Work out the finished part from the listing and answer in its coordinate system (mm). Face numbers are marked on the shaded views. Coordinates: 2 decimals unless noted, no trailing zeros. Loops run counter-clockwise (first coordinate to the right, second up) from the corner with the lowest first, then second, coordinate; pieces in that order, holes last. Notation, with made-up numbers: M -25.75,89 L 21.25,89 A16 ccw 21.25,105 Z; hole C 59,70 d5. An arc over 180 degrees is marked long. Write each question's results on one line, items separated by ' | '.
```python
from build123d import *

# Parameters (mm, degrees)
F1_DEPTH = 7
F2_DEPTH = 5
F3_W     = 25.4
F3_H     = 7
F4_DEPTH = 19.05
F6_DEPTH = 7


with BuildPart() as f1:
    # F0 (on Top) → F1 (new body)
    with BuildSketch(Plane.XY):
        with BuildLine():
            ThreePointArc((20, 20), (40, 0), (20, -20))
            Line((20, -20), (-40, -20))
            Line((-40, -20), (-40, -45.4))
            Line((-40, -45.4), (20, -45.4))
            ThreePointArc((20, -45.4), (65.4, 0), (20, 45.4))
            Line((20, 45.4), (-40, 45.4))
            Line((-40, 45.4), (-40, 20))
            Line((-40, 20), (20, 20))
        make_face()
        with BuildLine():
            Line((-40, -20), (20, -20))
            ThreePointArc((20, -20), (40, 0), (20, 20))
            Line((20, 20), (-40, 20))
            Line((-40, 20), (-40, -20))
        make_face()
    extrude(amount=F1_DEPTH)

    # F0 (on Top) → F2 (cut)
    with BuildSketch(Plane.XY):
        with BuildLine():
            Line((-40, -20), (20, -20))
            ThreePointArc((20, -20), (40, 0), (20, 20))
            Line((20, 20), (-40, 20))
            Line((-40, 20), (-40, -20))
        make_face()
    extrude(amount=F2_DEPTH, mode=Mode.SUBTRACT)

    # F3 (on face) → F4 (join)
    with BuildSketch(Plane(origin=(-40, 0, 0), x_dir=(0, -1, 0), z_dir=(-1, 0, 0))):
        with Locations((-32.7, 3.5)):
            Rectangle(F3_W, F3_H)
        with Locations((32.7, 3.5)):
            Rectangle(F3_W, F3_H)
    extrude(amount=F4_DEPTH)

    # F5 (on face) → F6 (join, through all)
    with BuildSketch(Plane(origin=(0, 0, 0), x_dir=(1, 0, 0), z_dir=(0, 0, -1))):
        with BuildLine():
            Line((-59.05, -65.72), (20, -65.72))
            ThreePointArc((20, -65.72), (85.72, 0), (20, 65.72))
            Line((20, 65.72), (-59.05, 65.72))
            Line((-59.05, 65.72), (-59.05, 45.4))
            Line((-59.05, 45.4), (20, 45.4))
            ThreePointArc((20, 45.4), (65.4, 0), (20, -45.4))
            Line((20, -45.4), (-59.05, -45.4))
            Line((-59.05, -45.4), (-59.05, -65.72))
        make_face()
    extrude(amount=-F6_DEPTH)


solid = f1.part
```
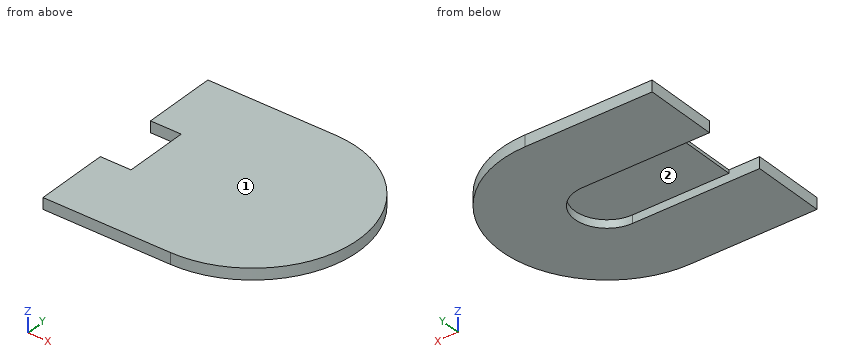
1) For a pull along Y with two mould halves and no side action, classify the marked faces 1 and 2 as released by +Y, released by -Y, zero draft, split by the parting line, or undercut.
Check result:
face 1: zero draft | face 2: undercut
2) Find section D-D, the plane y = 0. Give the vertices of the cut face in (x, z).
Check result:
outline: M -40,5 L 40,5 L 40,0 L 85.72,0 L 85.72,7 L -40,7 Z
3) Given pin 1 Ø1.5 at (x, z) = (49, 5.5) entering from +Y; pin 2 Ø2 at (x, y) = (49.5, 27) entering from -Z; pin 3 Ø2 at (y, z) = (6.5, 6.5) entering from -X, each flat-ended and moving along its own axis, determine where each tip first touches the part or whether it passes through.
Check result:
pin 1: y = 59.34 | pin 2: z = 0 | pin 3: x = -40
4) Straight lines are drawn through the part: probe 1 along Y at (x, z) = (7, 1); probe 2 along Y at (x, z) = (21.5, 2.25); probe 3 along Z at (x, y) = (25.5, -13). For each, find the intervals that lie inside material, in ascending order. Write a range as [from, to].
Check result:
probe 1: [-65.72, -20], [20, 65.72] | probe 2: [-65.7, -19.94], [19.94, 65.7] | probe 3: [5, 7]
5) Find section C-C, the plane x = 17.5. Give the vertices of the cut face in (y, z).
Check result:
outline: M -65.72,0 L -20,0 L -20,5 L 20,5 L 20,0 L 65.72,0 L 65.72,7 L -65.72,7 Z
6) Find section A-A, the plane x = -46. Give the vertices of the cut face in (y, z).
Check result:
outline: M -65.72,0 L -20,0 L -20,7 L -65.72,7 Z; M 20,0 L 65.72,0 L 65.72,7 L 20,7 Z
7) Find section B-B, the plane z = 2.25. Give the vertices of the cut face in (x, y), and give its area (3 significant figures).
Check result:
outline: M -59.05,-65.72 L 20,-65.72 A65.72 ccw 20,65.72 L -59.05,65.72 L -59.05,20 L 20,20 A20 cw 20,-20 L -59.05,-20 Z | area: 13,400 mm^2
